```python
from build123d import *

# Parameters (mm, degrees)
BOTTOM_FILLET_R = 0.4
FILLET1_R       = 0.6


with BuildPart() as part:
    # Sketch2 → Main Body (revolve)
    with BuildSketch(Plane(origin=(0, 0, 0), x_dir=(1, 0, 0), z_dir=(0, 1, 0))):
        with BuildLine():
            Line((2.1, 0), (5.35, 0))
            ThreePointArc((5.35, 0), (4.311757182, -3.167214865), (1.6, -5.105144464))
            Line((1.6, -5.105144464), (1.6, -3.319256268))
            Line((1.6, -3.319256268), (0.92, -3.319256268))
            Line((0.92, -3.319256268), (0.92, -2.149256268))
            ThreePointArc((0.92, -2.149256268), (1.782020191, -1.339298029), (2.1, -0.2))
            Line((2.1, -0.2), (2.1, 0))
        make_face()
    revolve(axis=Axis((0, 0, 0), (0, 0, 1)))

    # Bottom Fillet
    bottom_fillet_edges = [part.edges().sort_by_distance(p)[0] for p in [
        (-5.35, 0, 0),
        (-2.1, 0, 0),
    ]]
    fillet(bottom_fillet_edges, radius=BOTTOM_FILLET_R)

    # Fillet1
    fillet1_edges = [part.edges().sort_by_distance(p)[0] for p in [
        (-0.92, 0, 2.149256268),
    ]]
    fillet(fillet1_edges, radius=FILLET1_R)


solid = part.part
```
Work out the finished part from the listing and answer in its coordinate system (mm). Give positions to 0.01 mm unless a question says otherwise; leave off trailing zeros. Loops run counter-clockwise (first coordinate to the right, second up) from the corner with the lowest first, then second, coordinate; pieces in that order, holes last. Notation, with made-up numbers: (-12, 19) -> (46, 19) arc R31 cw to (46, 46) -> close; hole circle Ø4 at (71.25, -12). An arc over 180 degrees is marked (long way). Write item = value, one per line. Start each with the question number.
(1) Find section A-A on z = 3.05. Give the vertices of the cut face in (x, y), and give its area (3 significant figures).
(2) Given pin 1 Ø3 at (y, z) = (-1.5, 3.5) entering from +X; pin 2 Ø3.5 at (x, y) = (0.5, 0.5) entering from +Z; pin 3 Ø2 at (x, y) = (0, 0) entering from +Z; pin 4 Ø2.5 at (x, y) = (0, 0) entering from -Z, each flat-ended and moving along its own axis, determine where each tip first touches the part or whether it passes through.
(3) Find the intervals of material crossed by probe 1 along X at (y, z) = (0, 1); probe 2 along Y at (x, z) = (-1, 1.5); probe 3 along Y at (x, z) = (0, 4), in increasing order. Write a range as from..to.
(4) Find section B-B on z = 4.6. Give the vertices of the cut face in (x, y), and give its area (3 significant figures).
(5) The mould has two halves that part along Y. Classify faces 1 (the cylindrical face through (-1.27, -0.97, 4.2)), 2 (the cylindrical face through (0.878, 0.276, 2.896)), 3 (the flat face through (0, 3, 0)): +Y half, -Y half, draft (parallel to the pull), parting line (faces both ways), or undercut.
From the geometry:
q1.outline = circle Ø8.79 at (0, 0); hole circle Ø1.84 at (0, 0)
q1.area = 58.0 mm^2
q2.pin_1 = 4.83
q2.pin_2 = 5.11
q2.pin_3 = 3.32
q2.pin_4 = 1.94
q3.probe_1 = -5.26..-1.95, 1.95..5.26
q3.probe_2 = -5.04..-1.34, 1.34..5.04
q3.probe_3 = -3.55..-1.6, 1.6..3.55
q4.outline = circle Ø5.46 at (0, 0); hole circle Ø3.2 at (0, 0)
q4.area = 15.4 mm^2
q5.face_1 = undercut
q5.face_2 = undercut
q5.face_3 = draft
